Study the drawing (mm; zero at the part's minimum x, y, z) and answer. Coordinates: 2 decimals unless noted, no trailing zeros. Order: outer loops, then holes, each group sorted by start corner. A loop starts at its lowest first (then second) coordinate and runs counter-clockwise, first axis right, second up. Notation, with made-up numbers: M -39.5,13.5 L -2.5,13.5 A18 cw -2.5,23.5 Z; hole C 14.25,35 d4. An arc over 180 degrees is marked long. Use a Markdown table: item, result. Add a question column.
1) Find section C-C on y = 22. Write down the section's boundary in (x, z) (3 decimals).
2) Each of these flat-tipped pins is pushed along its axis until it touches: pin 1 Ø3.5 at (x, y) = (18, 2) entering from -Z; pin 2 Ø8 at (x, z) = (25.5, 40.5) entering from +Y; pin 3 Ø6 at (y, z) = (28, 20) entering from +X. Where does it stop, or does it pass through?
3) Find section B-B on x = 19.5. Write down the section's boundary in (y, z), plus the area to 3 significant figures.
4) Find the intervals of material crossed by probe 1 along Y at (x, z) = (1.9, 39.5); probe 2 along Y at (x, z) = (1.5, 31) (3 decimals); probe 3 along Y at (x, z) = (27, 2.5), in increasing order. Write a range as [from, to].
5) The mould has two halves that part along Y. Classify the marked faces 1, 2 and 3: released by +Y, released by -Y, zero draft, split by the parting line, or undercut.
6) Find section A-A on z = 15. Write down the section's boundary in (x, y) (3 decimals).
7) Find section D-D on z = 4. Write down the section's boundary in (x, y), plus the area to 3 significant figures.
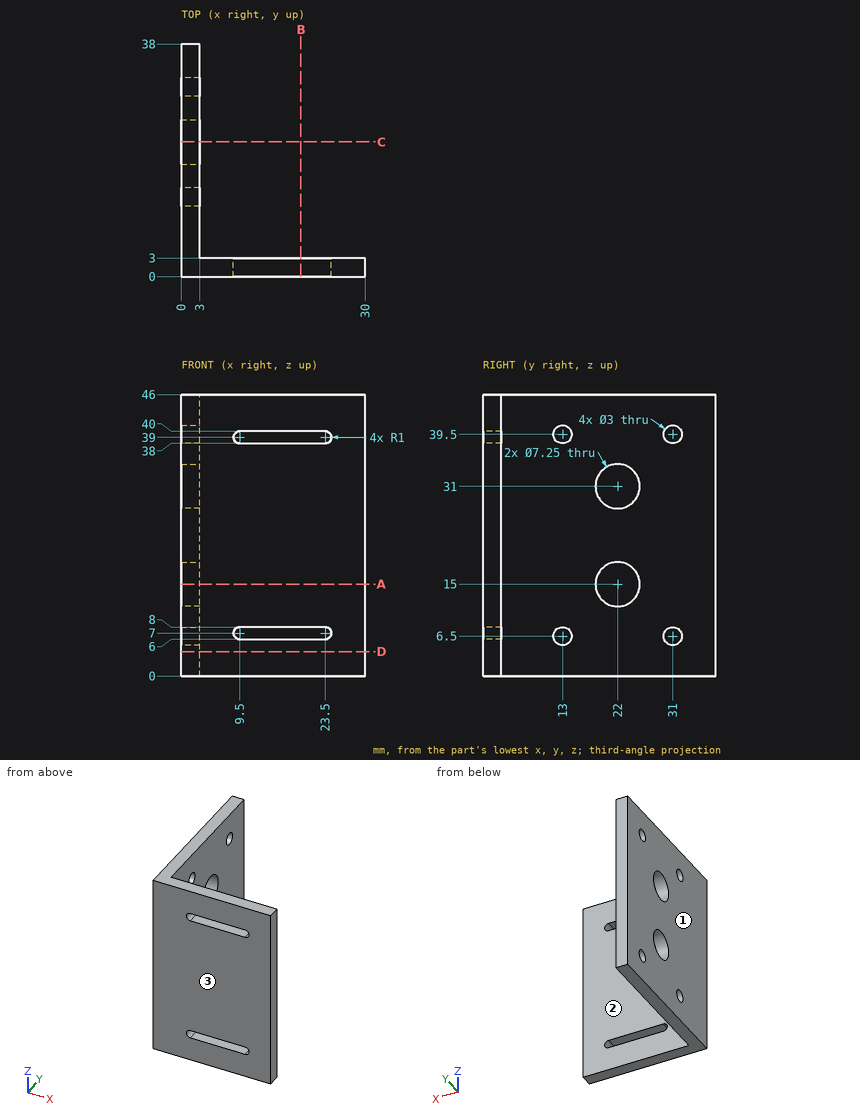
Check result:
| question | item | result |
|---|---|---|
| 1 | outline | M 0,0 L 3,0 L 3,11.375 L 0,11.375 Z; M 0,18.625 L 3,18.625 L 3,27.375 L 0,27.375 Z; M 0,34.625 L 3,34.625 L 3,46 L 0,46 Z |
| 2 | pin 1 | stops at z = 0 |
| 2 | pin 2 | stops at y = 3 |
| 2 | pin 3 | stops at x = 3 |
| 3 | outline | M 0,0 L 3,0 L 3,6 L 0,6 Z; M 0,8 L 3,8 L 3,38 L 0,38 Z; M 0,40 L 3,40 L 3,46 L 0,46 Z |
| 3 | area | 126 mm2 |
| 4 | probe 1 | y = [0, 11.5], [14.5, 29.5], [32.5, 38] |
| 4 | probe 2 | y = [0, 18.375], [25.625, 38] |
| 4 | probe 3 | y = [0, 3] |
| 5 | face 1 | zero draft |
| 5 | face 2 | released by +Y |
| 5 | face 3 | released by -Y |
| 6 | outline | M 0,0 L 30,0 L 30,3 L 3,3 L 3,18.375 L 0,18.375 Z; M 0,25.625 L 3,25.625 L 3,38 L 0,38 Z |
| 7 | outline | M 0,0 L 30,0 L 30,3 L 3,3 L 3,38 L 0,38 Z |
| 7 | area | 195 mm2 |
